from build123d import *

# Parameters (mm, degrees)
F1_DEPTH = 1


with BuildPart() as f1:
    # F0 (on Top) → F1 (new body)
    with BuildSketch(Plane.XY):
        with BuildLine():
            Line((58.383235, -101.68299), (70.444852, -88.32195))
            Line((70.444852, -88.32195), (64.843104, -71.005472))
            Line((64.843104, -71.005472), (63.735066, -67.580235))
            Line((63.735066, -67.580235), (58.133317, -50.263756))
            Line((58.133317, -50.263756), (40.531509, -46.498609))
            Line((40.531509, -46.498609), (39.903984, -49.432244))
            ThreePointArc((39.903984, -49.432244), (37.247557, -52.289482), (35.992471, -48.595544))
            Line((35.992471, -48.595544), (36.619996, -45.661909))
            Line((36.619996, -45.661909), (19.018187, -41.896762))
            Line((19.018187, -41.896762), (6.822551, -55.406257))
            Line((6.822551, -55.406257), (4.410228, -58.078465))
            Line((4.410228, -58.078465), (-7.785408, -71.587961))
            Line((-7.785408, -71.587961), (-2.245217, -88.714148))
            Line((-2.245217, -88.714148), (0.609147, -87.790783))
            ThreePointArc((0.609147, -87.790783), (4.411802, -88.662697), (1.840301, -91.596602))
            Line((1.840301, -91.596602), (-1.014064, -92.519967))
            Line((-1.014064, -92.519967), (4.526127, -109.646154))
            Line((4.526127, -109.646154), (22.323511, -113.453137))
            Line((22.323511, -113.453137), (25.843873, -114.206166))
            Line((25.843873, -114.206166), (43.641257, -118.013149))
            Line((43.641257, -118.013149), (55.702875, -104.65211))
            Line((55.702875, -104.65211), (53.476035, -102.64184))
            ThreePointArc((53.476035, -102.64184), (52.329808, -98.912687), (56.156395, -99.67272))
            Line((56.156395, -99.67272), (58.383235, -101.68299))
        make_face()
        with BuildLine():
            Line((4.410228, -58.078465), (6.822551, -55.406257))
            Line((6.822551, -55.406257), (4.521484, -53.328979))
            ThreePointArc((4.521484, -53.328979), (4.57471, -53.600792), (4.592551, -53.877193))
            ThreePointArc((4.592551, -53.877193), (3.839997, -55.511097), (2.10916, -56.001187))
            Line((2.10916, -56.001187), (4.410228, -58.078465))
        make_face()
        with BuildLine():
            ThreePointArc((4.592551, -53.877193), (4.57471, -53.600792), (4.521484, -53.328979))
            ThreePointArc((4.521484, -53.328979), (0.846649, -52.436499), (2.10916, -56.001187))
            ThreePointArc((2.10916, -56.001187), (3.839997, -55.511097), (4.592551, -53.877193))
        make_face()
        with BuildLine():
            ThreePointArc((66.684576, -66.626091), (66.311685, -68.638558), (67.792614, -70.051328))
            ThreePointArc((67.792614, -70.051328), (69.662763, -69.685116), (70.507313, -67.976813))
            ThreePointArc((70.507313, -67.976813), (69.073593, -65.949636), (66.684576, -66.626091))
        make_face()
        with BuildLine():
            Line((63.735066, -67.580235), (64.843104, -71.005472))
            Line((64.843104, -71.005472), (67.792614, -70.051328))
            ThreePointArc((67.792614, -70.051328), (66.311685, -68.638558), (66.684576, -66.626091))
            Line((66.684576, -66.626091), (63.735066, -67.580235))
        make_face()
        with BuildLine():
            Line((25.195431, -117.237589), (25.843873, -114.206166))
            Line((25.843873, -114.206166), (22.323511, -113.453137))
            Line((22.323511, -113.453137), (21.675069, -116.48456))
            ThreePointArc((21.675069, -116.48456), (23.639029, -115.908423), (25.195431, -117.237589))
        make_face()
        with BuildLine():
            ThreePointArc((25.339303, -118.010861), (25.303029, -117.61759), (25.195431, -117.237589))
            ThreePointArc((25.195431, -117.237589), (23.639029, -115.908423), (21.675069, -116.48456))
            ThreePointArc((21.675069, -116.48456), (22.362593, -119.995565), (25.339303, -118.010861))
        make_face()
    extrude(amount=F1_DEPTH)


solid = f1.part
Build history of the part. All positions in model axes, mm. A direction names the side the tool comes from. Round coordinates to 2 decimals unless told otherwise and drop trailing zeros. Write each loop counter-clockwise with the first axis right and the second up, starting at its lowest first coordinate (ties: lowest second). Pieces come first, ordered by that corner, then holes. Notation, with made-up numbers: M 81,-4 L 107,-4 A30 ccw 107,27 Z; hole C 17.5,10 d7. An arc over 180 degrees is marked long. Answer as a JSON object with one key per item and string values. Group by question number.
(1) Mould opens along X. For faces 5 (the cylindrical face through (0.89, -52.39, 0.49)), 6 (the flat face through (1.717, -100.963, 0.493)), 7 (the flat face through (34.618, -116.083, 0.493)), 8 (the flat face through (31, -80, 1)) say: pulls with the +X half, pulls with the -X half, needs draft (parallel to the pull), parting line crosses it, or undercut.
(2) Flat gauge pin, fed straight in: pin 1 (7.5 mm diameter, centred on x = 54.02, y = -100.44, fed in from +Z). Where does the tip first touch, or does it go through?
(3) Drill centre lines: L1, parallel to X at y = -66, z = 0.1; L2, parallel to X at y = -100.5, z = 0.3; L3, parallel to Y at x = 21.5, z = 0.45. Where is each one in solid material? Low to high.
(4) Which spindle directions (+Z, -Z, +X, -X, +Y, -Y) get a long thin tool onto all of the face, cutting with end or side? Do faces 1 (the flat face through (3.244, -57.025, 0.493)), 2 (the flat face through (5.688, -54.382, 0.493)), 3 (the flat face through (67.68, -79.78, 0.49)), 4 (the cylindrical face through (52.29, -98.96, 0.49)). Say none if no direction does.
(5) Cut at C-C (x = 20). Give the cut face in (y, z).
(6) Cut at B-B (y = -77). Give the cut face in (x, z), and give its area (3 significant figures).
Responses:
{
 "1": {"face 5": "undercut", "face 6": "pulls with the -X half", "face 7": "undercut", "face 8": "needs draft"},
 "2": {"pin 1": "stops at z = 1"},
 "3": {"L1": "x = -2.74 to 63.22, 67.51 to 69.2", "L2": "x = 1.57 to 51.75, 57.07 to 59.45", "L3": "y = -119.34 to -116.68, -113.28 to -42.43"},
 "4": {"face 1": "+Z, -Z, -X", "face 2": "+Z, -Z, +Y", "face 3": "+Z, -Z, +X", "face 4": "+Z, -Z"},
 "5": {"outline": "M -112.96,0 L -42.11,0 L -42.11,1 L -112.96,1 Z"},
 "6": {"outline": "M -6.03,0 L 66.78,0 L 66.78,1 L -6.03,1 Z", "area": "72.8 mm2"}
}
